```python
from build123d import *

# Parameters (mm, degrees)
SKETCH2_R                        = 3.15595
SKETCH2_R_2                      = 12.7
SKETCH2_R_3                      = 3.175
BOSS_EXTRUDE1_DEPTH              = 57.15
SKETCH3_W                        = 44.45
SKETCH3_H                        = 12.7
HOLLOWING_DEPTH                  = 25.4
FILLET2_R                        = 0.635
GEAR_CREVASE_DEPTH               = 6.477
SKETCH4_W                        = 57.15
SKETCH4_H                        = 25.4
BASE_EXTENSION_DEPTH             = 12.7
CAPTIVE_NUT_BORE_DEPTH           = 4.7625
HEX_CONNECTION_DEPTH             = 6.35
GEAR_CLEARANCE_DEPTH             = 6.477
BOSS_EXTRUDE6_DEPTH              = 6.35
BOSS_EXTRUDE7_START              = 50.8
BOSS_EXTRUDE7_DEPTH              = 6.35
SKETCH9_W                        = 9.6012
SKETCH9_H                        = 7.62
CUT_EXTRUDE5_DEPTH               = 11.43
CUT_EXTRUDE6_START               = -7.62
CUT_EXTRUDE6_DEPTH               = 7.62
F_10_0_1935_DIAMETER_HOLE1_D     = 5.0419
F_10_0_1935_DIAMETER_HOLE1_DEPTH = 7.62
FILLET3_R                        = 2.54
SKETCH14_R                       = 4.66725
CUT_EXTRUDE7_DEPTH               = 3.175


with BuildPart() as part:
    # Sketch2 → Boss-Extrude1 (new body)
    # profile 1 of 3: a face of its own
    with BuildSketch(Plane(origin=(0, 0, 0), x_dir=(0, 0, -1), z_dir=(1, 0, 0))):
        with BuildLine():
            Line((-12.994989453, 36.403030323), (0, 0))
            Line((0, 0), (0, 24.485346))
            Line((0, 24.485346), (-10.818105201, 37.636792682))
            ThreePointArc((-10.818105201, 37.636792682), (-11.256570169, 37.978374222), (-11.798913831, 38.1))
            ThreePointArc((-11.798913831, 38.1), (-12.83697729, 37.561658565), (-12.994989453, 36.403030323))
        make_face()
    # profile 2 of 3: a face of its own
    with BuildSketch(Plane(origin=(0, 0, 0), x_dir=(0, 0, -1), z_dir=(1, 0, 0))):
        with BuildLine():
            Line((0, 24.485346), (0, 0))
            Line((0, 0), (25.4, 0))
            Line((25.4, 0), (25.4, 25.4))
            ThreePointArc((25.4, 25.4), (12.7, 12.7), (0, 25.4))
            Line((0, 25.4), (0, 24.485346))
        make_face()
        with Locations((12.7, 9.525)):
            Circle(SKETCH2_R, mode=Mode.SUBTRACT)
    # profile 3 of 3: a face of its own
    with BuildSketch(Plane(origin=(0, 0, 0), x_dir=(0, 0, -1), z_dir=(1, 0, 0))):
        with Locations((12.7, 25.4)):
            Circle(SKETCH2_R_2)
        with Locations((12.7, 25.4)):
            Circle(SKETCH2_R_3, mode=Mode.SUBTRACT)
    extrude(amount=BOSS_EXTRUDE1_DEPTH)

    # Sketch3 → Hollowing (cut)
    with BuildSketch(Plane(origin=(0, 0, -25.4), x_dir=(-1, 0, 0), z_dir=(0, 0, -1))):
        Polygon((-50.8, 25.4), (-50.8, 15.875), (-31.8135, 15.875), (-31.8135, 0), (-25.3365, 0), (-25.3365, 15.875), (-6.35, 15.875), (-6.35, 25.4), align=None)
        with Locations((-28.575, 31.75)):
            Rectangle(SKETCH3_W, SKETCH3_H)
    extrude(amount=-HOLLOWING_DEPTH, mode=Mode.SUBTRACT)

    # Fillet2
    fillet2_edges = [part.edges().sort_by_distance(p)[0] for p in [
        (50.8, 15.875, -12.7),
        (25.3365, 15.875, -12.7),
        (31.8135, 15.875, -12.7),
        (6.35, 15.875, -12.7),
    ]]
    fillet(fillet2_edges, radius=FILLET2_R)

    # Sketch8 → Gear Crevase (add)
    with BuildSketch(Plane(origin=(25.3365, 0, 0), x_dir=(0, 0, -1), z_dir=(1, 0, 0))):
        with BuildLine():
            ThreePointArc((4.299739587, 0), (1.124739582, 4.299739599), (0, 9.525000025))
            Line((0, 9.525000025), (0, 0))
            Line((0, 0), (4.299739587, 0))
        make_face()
    extrude(amount=GEAR_CREVASE_DEPTH)

    # Sketch4 → Base Extension (add)
    with BuildSketch(Plane.XZ):
        with Locations((28.575, -12.7)):
            Rectangle(SKETCH4_W, SKETCH4_H)
    extrude(amount=BASE_EXTENSION_DEPTH)

    # Sketch7 → Captive Nut Bore (cut)
    with BuildSketch(Plane.ZY):
        Polygon((-9.470100522, 19.80565), (-6.240201043, 25.4), (-9.470100522, 30.99435), (-15.929899478, 30.99435), (-19.159798957, 25.4), (-15.929899478, 19.80565), align=None)
    extrude(amount=-CAPTIVE_NUT_BORE_DEPTH, mode=Mode.SUBTRACT)

    # Sketch5 → Hex Connection (add)
    with BuildSketch(Plane.XZ.offset(12.7)):
        Polygon((35.907348419, 0), (21.242651581, 0), (13.910303163, -12.7), (21.242651581, -25.4), (35.907348419, -25.4), (43.239696837, -12.7), align=None)
    extrude(amount=HEX_CONNECTION_DEPTH)

    # Sketch8<3> → Gear Clearance (cut)
    with BuildSketch(Plane(origin=(25.3365, 0, 0), x_dir=(0, 0, -1), z_dir=(1, 0, 0))):
        with BuildLine():
            Line((21.100260413, 0), (4.299739587, 0))
            ThreePointArc((4.299739587, 0), (12.7, -3.175), (21.100260413, 0))
        make_face()
    extrude(amount=GEAR_CLEARANCE_DEPTH, mode=Mode.SUBTRACT)

    # Sketch2<3> → Boss-Extrude6 (add)
    with BuildSketch(Plane(origin=(0, 0, 0), x_dir=(0, 0, -1), z_dir=(1, 0, 0))):
        with BuildLine():
            Line((-10.818105201, 37.636792682), (0, 24.485346))
            Line((0, 24.485346), (0, 25.4))
            ThreePointArc((0, 25.4), (3.719743879, 34.380256121), (12.7, 38.1))
            Line((12.7, 38.1), (-11.798913831, 38.1))
            ThreePointArc((-11.798913831, 38.1), (-11.256570169, 37.978374222), (-10.818105201, 37.636792682))
        make_face()
    extrude(amount=BOSS_EXTRUDE6_DEPTH)

    # Sketch2<4> → Boss-Extrude7 (add)
    with BuildSketch(Plane(origin=(0, 0, 0), x_dir=(0, 0, -1), z_dir=(1, 0, 0)).offset(BOSS_EXTRUDE7_START)):
        with BuildLine():
            Line((-10.818105201, 37.636792682), (0, 24.485346))
            Line((0, 24.485346), (0, 25.4))
            ThreePointArc((0, 25.4), (3.719743879, 34.380256121), (12.7, 38.1))
            Line((12.7, 38.1), (-11.798913831, 38.1))
            ThreePointArc((-11.798913831, 38.1), (-11.256570169, 37.978374222), (-10.818105201, 37.636792682))
        make_face()
    extrude(amount=BOSS_EXTRUDE7_DEPTH)

    # Sketch9 → Cut-Extrude5 (cut)
    with BuildSketch(Plane.XY):
        with Locations((28.575, -7.62)):
            Rectangle(SKETCH9_W, SKETCH9_H)
    extrude(amount=-CUT_EXTRUDE5_DEPTH, mode=Mode.SUBTRACT)

    # Sketch10 → Cut-Extrude6 (cut)
    with BuildSketch(Plane.XZ.offset(19.05).offset(CUT_EXTRUDE6_START)):
        Polygon((28.575, -7.156744595), (23.7744, -9.928372298), (23.7744, -15.471627702), (28.575, -18.243255405), (33.3756, -15.471627702), (33.3756, -9.928372298), align=None)
    extrude(amount=-CUT_EXTRUDE6_DEPTH, mode=Mode.SUBTRACT)

    # #10 (0.1935) Diameter Hole1
    with Locations(Plane(origin=(0, -19.05, 0), x_dir=(-1, 0, 0), z_dir=(0, -1, 0))):
        with Locations((-28.575, 12.7)):
            Hole(F_10_0_1935_DIAMETER_HOLE1_D / 2, depth=F_10_0_1935_DIAMETER_HOLE1_DEPTH)

    # Fillet3
    fillet3_edges = [part.edges().sort_by_distance(p)[0] for p in [
        (33.3756, -7.62, 0),
        (23.7744, -7.62, 0),
    ]]
    fillet(fillet3_edges, radius=FILLET3_R)

    # Sketch14 → Cut-Extrude7 (cut)
    with BuildSketch(Plane.ZY):
        with Locations((-12.7, 9.525)):
            Circle(SKETCH14_R)
    extrude(amount=-CUT_EXTRUDE7_DEPTH, mode=Mode.SUBTRACT)


solid = part.part
```
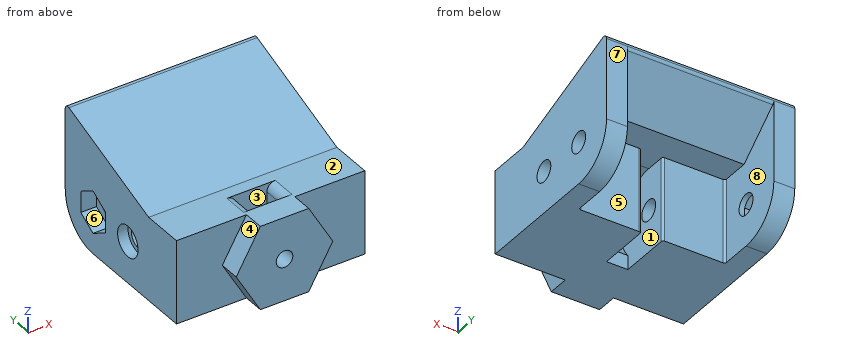
Input: part model. Units: mm. Frame: model coordinates. Face numbers are marked on the shaded views. A direction names the side the tool comes from. Give positions to 0.01 mm unless a question says otherwise; leave off trailing zeros. Order: outer loops, then holes, each group sorted by start corner. A loop starts at its lowest first (then second) coordinate and runs counter-clockwise, first axis right, second up. Notation, with made-up numbers: (89, 72.25) - (98, 72.25) arc R13 cw to (98, 87.25) - close; hole circle Ø3 at (76, -4.5). An arc over 180 degrees is marked (long way). Use a Markdown table: item, result.
(1) Access query for the marked faces 1, 2, 3, 4 and 5. Directions: +Z, -Z, +X, -X, +Y, -Y. A direction counts if a zero-diameter tool reaches every point of the face in a straight line with its end or side. Return the directions, or none.
Computed values:
| item | result |
|---|---|
| face 1 | +Y |
| face 2 | +Z, +X, -X, -Y |
| face 3 | +Z |
| face 4 | +Z, -X, -Y |
| face 5 | -Z, +Y |
(2) Line query: line 1 (Y direction, x = 1.9, z = -12.7); line 2 (Y direction, x = 5.5, z = -12.7) (3 decimals); line 3 (X direction, y = 21.5, z = -8). Output: solid intervals per line, ascending. Write a range as from..to.
Computed values:
| item | result |
|---|---|
| line 1 | y = -12.7..4.86, 14.19..19.81, 30.99..38.1 |
| line 2 | y = -12.7..6.369, 12.681..22.225, 28.575..38.1 |
| line 3 | x = 0..6.35, 50.8..57.15 |
(3) Draft query along Y for the marked faces 6, 7 and 8. Return one class per face: released by +Y, released by -Y, zero draft, split by the parting line, or undercut.
Computed values:
| item | result |
|---|---|
| face 6 | undercut |
| face 7 | released by +Y |
| face 8 | zero draft |
(4) Pin query (flat end, axial travel): pin 1 (7.5 mm diameter, centred on x = 26.5, z = -9.5, fed in from +Y) (3 decimals); pin 2 (6 mm diameter, centred on x = 28.575, z = -12.7, fed in from +Y); pin 3 (4.5 mm diameter, centred on y = 10.5, z = -11, fed in from -X) (3 decimals); pin 4 (4 mm diameter, centred on y = 9.525, z = -12.7, fed in from -X). Return the tip coordinate at first contact, or that it passes through.
Computed values:
| item | result |
|---|---|
| pin 1 | stops at y = 15.875 |
| pin 2 | stops at y = -2.82 |
| pin 3 | stops at x = 3.175 |
| pin 4 | passes through |
(5) Section query A-A (x = 54). Output: boundary loops of the cut face in (y, z) (3 decimals).
Computed values:
| item | result |
|---|---|
| outline | (-12.7, -25.4) - (25.4, -25.4) arc R12.7 ccw to (38.1, -12.7) - (38.1, 11.799) arc R1.27 ccw to (36.403, 12.995) - (0, 0) - (-12.7, 0) - close; hole circle Ø6.312 at (9.525, -12.7); hole circle Ø6.35 at (25.4, -12.7) |
(6) Section query B-B (x = 11). Output: boundary loops of the cut face in (y, z) (3 decimals), then the cut area to 3 significant figures.
Computed values:
| item | result |
|---|---|
| outline | (-12.7, -25.4) - (15.875, -25.4) - (15.875, 0) - (24.485, 0) - (37.637, 10.818) arc R1.27 ccw to (36.403, 12.995) - (0, 0) - (-12.7, 0) - close; hole circle Ø6.312 at (9.525, -12.7) |
| area | 877 mm2 |
(7) Section query C-C (y = 11). State how many separate pieces and enclosed holes the cut face has, then the cut area to 3 significant figures.
Computed values:
| item | result |
|---|---|
| separate pieces | 3 |
| enclosed holes | 0 |
| area | 1,220 mm2 |
